Model file for the job. Use its own axes, mm. Give positions to 0.01 mm unless a question says otherwise; leave off trailing zeros. Order: outer loops, then holes, each group sorted by start corner. A loop starts at its lowest first (then second) coordinate and runs counter-clockwise, first axis right, second up. Notation, with made-up numbers: (10.25, -5) - (41.25, -5) arc R9 ccw to (41.25, 0) - close; hole circle Ø9 at (64, 16.25). An arc over 180 degrees is marked (long way). Use CSV: the item, a comma, the result in double quotes. Start each with the question number.
(1) Drop flat-ended pins along their axis: pin 1 Ø1.5 at (x, z) = (0.5, 5.5) entering from +Y; pin 2 Ø4 at (x, y) = (-44.5, 0) entering from +Z. Give the stop position or say it passes through.
(2) Probe L1, parallel to X at y = 43, z = 0.75; L2, parallel to X at y = 12, z = 1.5; L3, parallel to Y at x = -44.5, z = 4.5. List the from-to ranges inside material, lowest first.
(3) Band-saw the part on A-A, the plane z = 3.5. Count the separate pieces of the cut face and the enclosed holes in it, then the cut area to 3 significant figures.
(4) Band-saw the part on B-B, the plane x = 17. Give the cut face in (y, z), then the cut area to 3 significant figures.
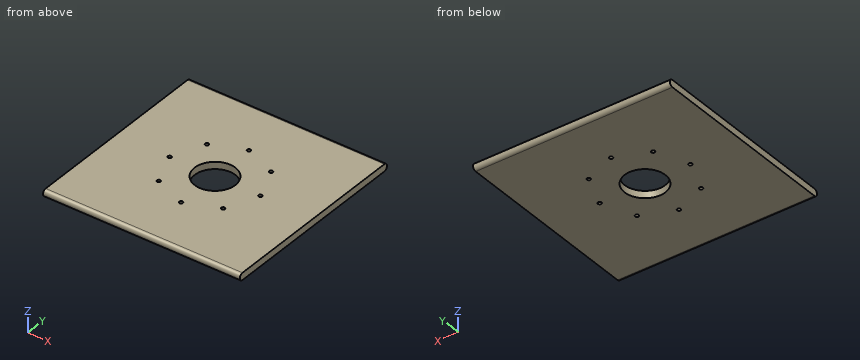
from build123d import *

# Parameters (mm, degrees)
SKETCH_1_W          = 193
SKETCH_1_H          = 193
EXTRUDE_1_DEPTH     = 7
SKETCH_2_R          = 20
CUT_EXTRUDE_1_DEPTH = 123
SKETCH_3_R          = 1.75
CUT_EXTRUDE_2_DEPTH = 137.651015364
FILLET_2_RADIUS     = 3.5
FILLET_2_LENGTH     = 193
FILLET_4_RADIUS     = 3.5
FILLET_4_LENGTH     = 193


with BuildPart() as part:
    # 草图1 → 凸台-拉伸1 (new body)
    with BuildSketch(Plane.XY):
        Rectangle(SKETCH_1_W, SKETCH_1_H)
    extrude(amount=EXTRUDE_1_DEPTH)

    # 草图2 → 切除-拉伸1 (cut)
    with BuildSketch(Plane.XY.offset(7)):
        Circle(SKETCH_2_R)
    extrude(amount=-CUT_EXTRUDE_1_DEPTH, mode=Mode.SUBTRACT)

    # 草图3 → 切除-拉伸2 (cut, through all)
    with BuildSketch(Plane.XY.offset(7)):
        with Locations((0, 44.5)):
            Circle(SKETCH_3_R)
        with Locations((31.466251763, 31.466251763)):
            Circle(SKETCH_3_R)
        with Locations((44.5, 0)):
            Circle(SKETCH_3_R)
        with Locations((31.466251763, -31.466251763)):
            Circle(SKETCH_3_R)
        with Locations((0, -44.5)):
            Circle(SKETCH_3_R)
        with Locations((-31.466251763, -31.466251763)):
            Circle(SKETCH_3_R)
        with Locations((-44.5, 0)):
            Circle(SKETCH_3_R)
        with Locations((-31.466251763, 31.466251763)):
            Circle(SKETCH_3_R)
    extrude(amount=-CUT_EXTRUDE_2_DEPTH, mode=Mode.SUBTRACT)

    # 圆角2: full round fillet: the end face becomes a half cylinder, R = half its width
    fillet_2_face = Plane((0, 96.5, 3.5), x_dir=(-1, 0, 0), z_dir=(0, 1, 0))  # on the end face: x along it, z out of the body
    fillet_2_slab = fillet_2_face.offset(-FILLET_2_RADIUS / 2) * Box(FILLET_2_LENGTH, 2 * FILLET_2_RADIUS, FILLET_2_RADIUS, mode=Mode.PRIVATE)  # the body's end, R deep
    fillet_2_round = Plane((0, 93, 3.5), x_dir=(0, 1, 0), z_dir=(-1, 0, 0)) * Cylinder(FILLET_2_RADIUS, FILLET_2_LENGTH, mode=Mode.PRIVATE)  # its axis R under the face
    add(fillet_2_slab - fillet_2_round, mode=Mode.SUBTRACT)

    # 圆角4: full round fillet: the end face becomes a half cylinder, R = half its width
    fillet_4_face = Plane((0, -96.5, 3.5), x_dir=(-1, 0, 0), z_dir=(0, -1, 0))  # on the end face: x along it, z out of the body
    fillet_4_slab = fillet_4_face.offset(-FILLET_4_RADIUS / 2) * Box(FILLET_4_LENGTH, 2 * FILLET_4_RADIUS, FILLET_4_RADIUS, mode=Mode.PRIVATE)  # the body's end, R deep
    fillet_4_round = Plane((0, -93, 3.5), x_dir=(0, -1, 0), z_dir=(-1, 0, 0)) * Cylinder(FILLET_4_RADIUS, FILLET_4_LENGTH, mode=Mode.PRIVATE)  # its axis R under the face
    add(fillet_4_slab - fillet_4_round, mode=Mode.SUBTRACT)


solid = part.part
Answer block:
1,pin 1,"stops at y = 96.27"
1,pin 2,"stops at z = 7"
2,L1,"x = -96.5 to -0.9, 0.9 to 96.5"
2,L2,"x = -96.5 to -16, 16 to 96.5"
2,L3,"y = -96.35 to -1.75, 1.75 to 96.35"
3,separate pieces,"1"
3,enclosed holes,"9"
3,area,"35,900 mm2"
4,outline,"(-93, 0) - (-10.54, 0) - (-10.54, 7) - (-93, 7) arc R3.5 ccw to start; (10.54, 0) - (93, 0) arc R3.5 ccw to (93, 7) - (10.54, 7) - close"
4,area,"1,190 mm2"
